Autodesk Fusion 360 part; units mm, degrees
sketch "草图1" plane through (0, 0, 0) normal (0, 1, 0) x (1, 0, 0)
  line L0 (0, -6) -> (9, -6)
  line L1 (9, -6) -> (9, 18)
  line L2 (9, 18) -> (0, 18)
  line L3 (0, 18) -> (0, -6)
extrude "拉伸1" add sketch "草图1" along normal blind 5 and the other way blind 0
extrude "拉伸2" add 1 faces at (3, 5, -10) along direction (0, 1, 0) blind 5
cylinder "圆柱体基本要素1" add diameter 3 height 9 placed x (0, 0, -1) y (0, 1, 0) z (1, 0, 0) at (9, 5, 0)
cylinder "圆柱体基本要素2" add diameter 38 height 27 placed x (0, 0, -1) y (0, 1, 0) z (1, 0, 0) at (18, 5, 0)
Input: part model. Units: mm. Frame: model coordinates. A direction names the side the tool comes from. Give positions to 0.01 mm unless a question says otherwise; leave off trailing zeros. Write each loop counter-clockwise with the first axis right and the second up, starting at its lowest first coordinate (ties: lowest second). Pieces come first, ordered by that corner, then holes. Notation, with made-up numbers: M 68.25,34 L 101.25,34 A14 ccw 101.25,55 Z; hole C 26,-34.75 d11. An arc over 180 degrees is marked long. Write item = value, one per line. Start each with the question number.
1) Cut plane C-C on z = 0. Return the cut outline in (x, y).
2) First-contact query: pin 1 Ø12 at (x, y) = (35, 18.5) entering from +Z; pin 2 Ø7 at (x, z) = (4.5, -1.5) entering from -Y; pin 3 Ø2 at (x, z) = (30, 14.5) entering from +Y; pin 4 Ø3 at (x, y) = (16, 17) entering from +Z. Flat tips, straight axial feed; report the tip coordinate or a pass-through.
3) Cut plane A-A on z = -5. Return the cut outline in (x, y), then the cut area to 3 significant figures.
4) Cut plane B-B on y = 5. Return the cut outline in (x, z), then the cut area to 3 significant figures.
5) Material intervals for line 1 along X through (y, z) = (18, -1); line 2 along X through (y, z) = (3, -0.5); line 3 along Y through (x, z) = (25, 0.5), sorted ascending. Write a range as [from, to].
6) Cut plane D-D on z = -15.5. Return the cut outline in (x, y).
7) Reachability of faces 1 (the flat face through (5, 5, -18)), 2 (the cylindrical face through (13.56, 5.07, 1.5)), 3 (the flat face through (4, 0, -6)), 4 (the flat face through (4, 10, -6)) from +Z, -Z, +X, -X, +Y, -Y: full face, straight path, thin tool, end or side. Return the list, or none.
Solved:
q1.outline = M 0,0 L 9,0 L 9,3.5 L 18,3.5 L 18,-14 L 45,-14 L 45,24 L 18,24 L 18,6.5 L 9,6.5 L 9,10 L 0,10 Z
q2.pin_1 = 17.46
q2.pin_2 = 0
q2.pin_3 = 18.37
q2.pin_4 = through
q3.outline = M 0,0 L 9,0 L 9,10 L 0,10 Z; M 18,-13.33 L 45,-13.33 L 45,23.33 L 18,23.33 Z
q3.area = 1,080 mm2
q4.outline = M 0,-18 L 9,-18 L 9,-1.5 L 18,-1.5 L 18,-19 L 45,-19 L 45,19 L 18,19 L 18,1.5 L 9,1.5 L 9,6 L 0,6 Z
q4.area = 1,270 mm2
q5.line_1 = [18, 45]
q5.line_2 = [0, 9], [18, 45]
q5.line_3 = [-13.99, 23.99]
q6.outline = M 0,0 L 9,0 L 9,10 L 0,10 Z; M 18,-5.99 L 45,-5.99 L 45,15.99 L 18,15.99 Z
q7.face_1 = -Z, -X, +Y, -Y
q7.face_2 = none
q7.face_3 = +Z, -Z, -X, -Y
q7.face_4 = +Z, -Z, -X, +Y
